Can you work these out from the model? Positions are in its coordinate system, mm. Round coordinates to 2 decimals unless told otherwise and drop trailing zeros. Loops run counter-clockwise (first coordinate to the right, second up) from the corner with the lowest first, then second, coordinate; pieces in that order, holes last. Notation, with made-up numbers: (-5.5, 37.25) -> (1.5, 37.25) arc R15 cw to (1.5, 46.25) -> close; hole circle Ø11 at (89, 37.5). An arc over 180 degrees is marked (long way). Use a Markdown table: item, result.
from build123d import *

# Parameters (mm, degrees)
F1_DEPTH      = 13
F1_DEPTH_BACK = 13
F2_R          = 10


with BuildPart() as f1:
    # F0 (on Front) → F1 (new body, two sides)
    with BuildSketch(Plane.XZ) as f1_sk:
        Polygon((-53.997823, -24.075741), (-39.376436, -24.075741), (-34.858179, -10.169976), (-46.687129, -1.575741), (-58.516079, -10.169976), align=None)
    extrude(amount=F1_DEPTH)
    extrude(f1_sk.sketch, amount=-F1_DEPTH_BACK)

    # F2
    f2_edges = [f1.edges().sort_by_distance(p)[0] for p in [
        (-52.601604, -13, -5.872858),
        (-56.256951, -13, -17.122858),
        (-46.687129, -13, -24.075741),
        (-37.117308, -13, -17.122858),
        (-40.772654, -13, -5.872858),
        (-52.601604, 13, -5.872858),
        (-56.256951, 13, -17.122858),
        (-46.687129, 13, -24.075741),
        (-37.117308, 13, -17.122858),
        (-40.772654, 13, -5.872858),
    ]]
    fillet(f2_edges, radius=F2_R)


solid = f1.part
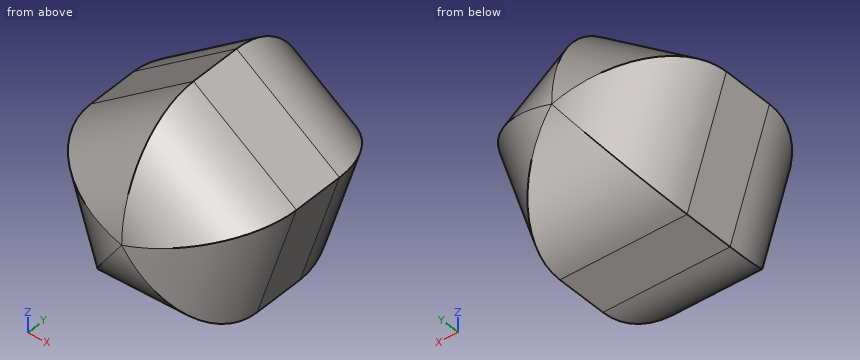
1. Will these pins go through, and if not, where does the flat tip stop? pin 1 Ø3 at (x, y) = (-41, 7.5) entering from +Z; pin 2 Ø1 at (y, z) = (-1, -19) entering from +X; pin 3 Ø3 at (x, y) = (-52, 7) entering from +Z.
Answer sheet:
| item | result |
|---|---|
| pin 1 | stops at z = -5.66 |
| pin 2 | stops at x = -37.56 |
| pin 3 | stops at z = -5.16 |
2. I need wall thicknesses on line 1 (X direction, y = 8, z = -19.75); line 2 (X direction, y = 9.75, z = -8.25); line 3 (Y direction, x = -51, z = -11). Which ranges of each line are inside material? Lowest first, please.
Answer sheet:
| item | result |
|---|---|
| line 1 | x = -53.99 to -39.38 |
| line 2 | x = -51.41 to -41.96 |
| line 3 | y = -11.71 to 11.71 |
3. I want a section at A-A (y = 1.75). Please give me the cut outline in (x, z).
Answer sheet:
| item | result |
|---|---|
| outline | (-58.52, -10.17) -> (-54, -24.08) -> (-39.38, -24.08) -> (-34.86, -10.17) -> (-46.69, -1.58) -> close |
4. I want a section at B-B (y = 8). Please give me the cut outline in (x, z), plus the area to 3 significant figures.
Answer sheet:
| item | result |
|---|---|
| outline | (-56.94, -10.68) -> (-53.02, -22.74) -> (-40.35, -22.74) -> (-36.43, -10.68) -> (-46.69, -3.23) -> close |
| area | 276 mm² |
